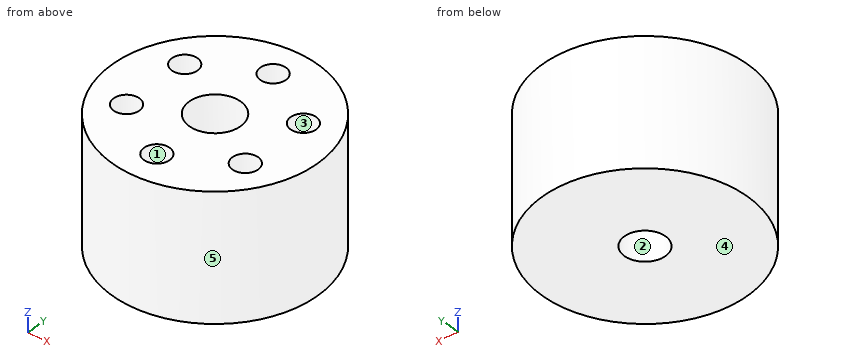
```python
from build123d import *

# Parameters (mm, degrees)
SKETCH_1_R          = 20
EXTRUDE_1_DEPTH     = 24.5
SKETCH_2_R          = 5
CUT_EXTRUDE_1_DEPTH = 10
SKETCH_3_R          = 4
CUT_EXTRUDE_2_DEPTH = 32.784430151
SKETCH_4_R          = 2.5
CUT_EXTRUDE_3_DEPTH = 10


with BuildPart() as part:
    # 스케치1 → 보스-돌출1 (new body)
    with BuildSketch(Plane.XY):
        Circle(SKETCH_1_R)
    extrude(amount=EXTRUDE_1_DEPTH)

    # 스케치2 → 컷-돌출1 (cut)
    with BuildSketch(Plane.XY.offset(24.5)):
        Circle(SKETCH_2_R)
    extrude(amount=-CUT_EXTRUDE_1_DEPTH, mode=Mode.SUBTRACT)

    # 스케치3 → 컷-돌출2 (cut, through all)
    with BuildSketch(Plane.XY.offset(14.5)):
        Circle(SKETCH_3_R)
    extrude(amount=-CUT_EXTRUDE_2_DEPTH, mode=Mode.SUBTRACT)

    # 스케치4 → 컷-돌출3 (cut)
    with BuildSketch(Plane.XY.offset(24.5)):
        with Locations((11.691342951, 6.75)):
            Circle(SKETCH_4_R)
        with Locations((0, 13.5)):
            Circle(SKETCH_4_R)
        with Locations((11.691342951, -6.75)):
            Circle(SKETCH_4_R)
        with Locations((0, -13.5)):
            Circle(SKETCH_4_R)
        with Locations((-11.691342951, -6.75)):
            Circle(SKETCH_4_R)
        with Locations((-11.691342951, 6.75)):
            Circle(SKETCH_4_R)
    extrude(amount=-CUT_EXTRUDE_3_DEPTH, mode=Mode.SUBTRACT)


solid = part.part
```
Could you check a few things on this model? Use its own coordinates, in mm. Face numbers are marked on the shaded views. A direction names the side the tool comes from. Give positions to 0.01 mm unless a question says otherwise; leave off trailing zeros. Loops run counter-clockwise (first coordinate to the right, second up) from the corner with the lowest first, then second, coordinate; pieces in that order, holes last. Notation, with made-up numbers: (58, 5.5) -> (102, 5.5) arc R9 cw to (102, 19.5) -> close; hole circle Ø6 at (86.5, 47.25). An arc over 180 degrees is marked (long way). Put each result on its own line as item: value.
(1) Imagine slicing it at D-D on y = -13.5. Write out the boundary of the cut face in (x, z), plus the area to 3 significant figures.
Computed:
outline: (-14.76, 0) -> (14.76, 0) -> (14.76, 24.5) -> (2.5, 24.5) -> (2.5, 14.5) -> (-2.5, 14.5) -> (-2.5, 24.5) -> (-14.76, 24.5) -> close
area: 673 mm^2
(2) Please list where these lines run through material, in increasing order: probe 1 along Y at (x, z) = (0, 22); probe 2 along Y at (x, z) = (13, 17.75); probe 3 along X at (y, z) = (8.5, 19.75). Write a range as [from, to].
Computed:
probe 1: [-20, -16], [-11, -5], [5, 11], [16, 20]
probe 2: [-15.2, -8.88], [-4.62, 4.62], [8.88, 15.2]
probe 3: [-18.1, -13.48], [-9.91, 9.91], [13.48, 18.1]
(3) Imagine slicing it at C-C on x = 0. Write out the boundary of the cut face in (y, z), plus the area to 3 significant figures.
Computed:
outline: (-20, 0) -> (-4, 0) -> (-4, 14.5) -> (-5, 14.5) -> (-5, 24.5) -> (-11, 24.5) -> (-11, 14.5) -> (-16, 14.5) -> (-16, 24.5) -> (-20, 24.5) -> close; (4, 0) -> (20, 0) -> (20, 24.5) -> (16, 24.5) -> (16, 14.5) -> (11, 14.5) -> (11, 24.5) -> (5, 24.5) -> (5, 14.5) -> (4, 14.5) -> close
area: 664 mm^2
(4) Imagine slicing it at A-A on y = 0. Write out the boundary of the cut face in (x, z), plus the area to 3 significant figures.
Computed:
outline: (-20, 0) -> (-4, 0) -> (-4, 14.5) -> (-5, 14.5) -> (-5, 24.5) -> (-20, 24.5) -> close; (4, 0) -> (20, 0) -> (20, 24.5) -> (5, 24.5) -> (5, 14.5) -> (4, 14.5) -> close
area: 764 mm^2
(5) Thinking about a two-plate mould opening in X: for the marked faces 3, 4 and 5, which applies, pulls with the +X half, pulls with the -X half, needs draft (parallel to the pull), parting line crosses it, or undercut?
Computed:
face 3: undercut
face 4: needs draft
face 5: parting line crosses it
(6) I'm going to push flat-ended pins straight in: pin 1 Ø2 at (x, z) = (8.5, 17) entering from -Y; pin 2 Ø10 at (x, z) = (-4.5, 18) entering from +Y; pin 3 Ø2.5 at (x, y) = (11, 6.5) entering from +Z; pin 4 Ø6.5 at (x, y) = (0, 0) entering from -Z. Where does each tip first touch, or does it pass through?
Computed:
pin 1: y = -18.54
pin 2: y = 20
pin 3: z = 14.5
pin 4: through
(7) Imagine slicing it at B-B on z = 21.5. Write out the boundary of the cut face in (x, y), plus the area to 3 significant figures.
Computed:
outline: circle Ø40 at (0, 0); hole circle Ø5 at (-11.69, -6.75); hole circle Ø5 at (-11.69, 6.75); hole circle Ø10 at (0, 0); hole circle Ø5 at (0, -13.5); hole circle Ø5 at (0, 13.5); hole circle Ø5 at (11.69, -6.75); hole circle Ø5 at (11.69, 6.75)
area: 1,060 mm^2
(8) For the marked faces 1 and 2, which set-ups out of +Z, -Z, +X, -X, +Y, -Y let a thin tool reach every point of the face, with its end or its side?
Computed:
face 1: +Z
face 2: +Z, -Z
